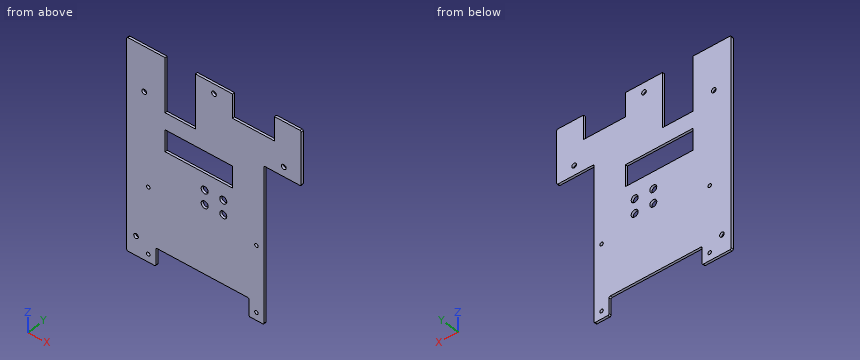
from build123d import *

# Parameters (mm, degrees)
CROQUIS1_W         = 150
CROQUIS1_H         = 175.2
CROQUIS1_R         = 1.5
EXTRUIR1_DEPTH     = 2
CROQUIS2_W         = 80
CROQUIS2_H         = 15
EXTRUIR2_DEPTH     = 10
CROQUIS3_W         = 32
CROQUIS3_H         = 130
EXTRUIR3_DEPTH     = 10
CROQUIS4_R         = 2
EXTRUIR4_DEPTH     = 10
CROQUIS5_R         = 3
EXTRUIR5_DEPTH     = 10
MATRIZL1_COUNT     = 2
MATRIZL1_PITCH     = 8
MATRIZL1_COL_COUNT = 2
MATRIZL1_COL_PITCH = 8
CROQUIS6_R         = 3
EXTRUIR6_DEPTH     = 2
CROQUIS7_W         = 26
CROQUIS7_H         = 45.2
CROQUIS7_W_2       = 36
CROQUIS7_H_2       = 20
CROQUIS7_W_3       = 58
CROQUIS7_H_3       = 18
EXTRUIR7_DEPTH     = 10
REDONDEO1_R        = 1


with BuildPart() as part:
    # Croquis1 → Extruir1 (new body)
    with BuildSketch(Plane(origin=(0, 0, 0), x_dir=(1, 0, 0), z_dir=(0, 1, 0))):
        Rectangle(CROQUIS1_W, CROQUIS1_H)
        with Locations(Location((-56.5, 81.1, 0), (0, 0, 270))):
            Circle(CROQUIS1_R, mode=Mode.SUBTRACT)
        with Locations(Location((36.5, 81.1, 0), (0, 0, 270))):
            Circle(CROQUIS1_R, mode=Mode.SUBTRACT)
        with Locations(Location((-56.5, 26.1, 0), (0, 0, 270))):
            Circle(CROQUIS1_R, mode=Mode.SUBTRACT)
        with Locations(Location((36.5, 26.1, 0), (0, 0, 270))):
            Circle(CROQUIS1_R, mode=Mode.SUBTRACT)
    extrude(amount=EXTRUIR1_DEPTH)

    # Croquis2 → Extruir2 (cut)
    with BuildSketch(Plane(origin=(0, 2, 0), x_dir=(1, 0, 0), z_dir=(0, 1, 0))):
        with Locations((-10, 80.1)):
            Rectangle(CROQUIS2_W, CROQUIS2_H)
    extrude(amount=-EXTRUIR2_DEPTH, mode=Mode.SUBTRACT)

    # Croquis3 → Extruir3 (cut)
    with BuildSketch(Plane(origin=(0, 2, 0), x_dir=(1, 0, 0), z_dir=(0, 1, 0))):
        with Locations((59, 22.6)):
            Rectangle(CROQUIS3_W, CROQUIS3_H)
    extrude(amount=-EXTRUIR3_DEPTH, mode=Mode.SUBTRACT)

    # Croquis4 → Extruir4 (cut)
    with BuildSketch(Plane(origin=(0, 2, 0), x_dir=(1, 0, 0), z_dir=(0, 1, 0))):
        with Locations(Location((-60, -50.4, 0), (0, 0, 270))):
            Circle(CROQUIS4_R)
        with Locations(Location((60, -50.4, 0), (0, 0, 270))):
            Circle(CROQUIS4_R)
        with Locations(Location((-67, 71.6, 0), (0, 0, 270))):
            Circle(CROQUIS4_R)
        with Locations(Location((0, -79.6, 0), (0, 0, 270))):
            Circle(CROQUIS4_R)
    extrude(amount=-EXTRUIR4_DEPTH, mode=Mode.SUBTRACT)

    # Croquis5 → Extruir5 (cut)
    with BuildSketch(Plane(origin=(0, 2, 0), x_dir=(1, 0, 0), z_dir=(0, 1, 0))):
        with Locations(Location((0, 15.6, 0), (0, 0, 270))):
            Circle(CROQUIS5_R)
        with Locations(Location((0, 3.6, 0), (0, 0, 270))):
            Circle(CROQUIS5_R)
    extruir5 = extrude(amount=-EXTRUIR5_DEPTH, mode=Mode.SUBTRACT)

    # MatrizL1: Extruir5 ×2
    with Locations(*[(-i * MATRIZL1_PITCH, 0, 0) for i in range(1, MATRIZL1_COUNT)]):
        add(extruir5, mode=Mode.SUBTRACT)

    # MatrizL1 col: Extruir5 ×2
    with Locations(*[(i * MATRIZL1_COL_PITCH, 0, 0) for i in range(1, MATRIZL1_COL_COUNT)]):
        add(extruir5, mode=Mode.SUBTRACT)

    # Croquis6 → Extruir6 (add)
    with BuildSketch(Plane(origin=(0, 2, 0), x_dir=(1, 0, 0), z_dir=(0, 1, 0))):
        with Locations((0, 15.6)):
            Circle(CROQUIS6_R)
        with Locations((0, 3.6)):
            Circle(CROQUIS6_R)
    extrude(amount=-EXTRUIR6_DEPTH)

    # Croquis7 → Extruir7 (cut)
    with BuildSketch(Plane(origin=(0, 2, 0), x_dir=(1, 0, 0), z_dir=(0, 1, 0))):
        with Locations((-29, -65)):
            Rectangle(CROQUIS7_W, CROQUIS7_H)
        with Locations((34, -77.6)):
            Rectangle(CROQUIS7_W_2, CROQUIS7_H_2)
        with Locations((-13, -19.4)):
            Rectangle(CROQUIS7_W_3, CROQUIS7_H_3)
    extrude(amount=-EXTRUIR7_DEPTH, mode=Mode.SUBTRACT)

    # Redondeo1
    redondeo1_edges = [part.edges().sort_by_distance(p)[0] for p in [
        (30, 1, -87.6),
        (-50, 1, -87.6),
        (30, 1, -72.6),
        (-50, 1, -72.6),
        (43, 1, -87.6),
        (75, 1, 42.4),
        (43, 1, 42.4),
        (-75, 1, -87.6),
        (75, 1, 87.6),
        (-75, 1, 87.6),
    ]]
    fillet(redondeo1_edges, radius=REDONDEO1_R)


solid = part.part
Source: CAD feature listing. Evaluate the final solid. Frame: model axes, mm. Round coordinates to 2 decimals unless told otherwise and drop trailing zeros. Loops run counter-clockwise (first coordinate to the right, second up) from the corner with the lowest first, then second, coordinate; pieces in that order, holes last.
Q1. Section A-A, the plane x = 0. Return loops of the section in (y, z), plus the area to 3 significant figures.
Q2. Section C-C, the plane x = -60. Return loops of the section in (y, z).
Q3. First-contact query: P1, Ø5, axis at x = 36.5, z = -81.1, coming from the +Y side; P2, Ø1, axis at x = 62, y = 1, coming from the -Z side. Flat tips, straight axial feed; report the tip coordinate or a pass-through.
Q4. Ray query, line 1 (X direction, y = 1.25, z = -81.1); line 2 (X direction, y = 0.9, z = -3.6); line 3 (Z direction, x = 7.5, y = 1.9). Return the intervals inside material, ascending.
Q5. Section B-B, the plane z = -15.6. Return loops of the section in (x, y).
Q6. Section D-D, the plane z = 65.5. Return loops of the section in (x, y), plus the area to 3 significant figures.
Solutions:
1. outline: (0, -72.6) - (2, -72.6) - (2, 10.4) - (0, 10.4) - close; (0, 28.4) - (2, 28.4) - (2, 77.6) - (0, 77.6) - close; (0, 81.6) - (2, 81.6) - (2, 87.6) - (0, 87.6) - close
1. area: 276 mm2
2. outline: (0, -87.6) - (2, -87.6) - (2, 48.4) - (0, 48.4) - close; (0, 52.4) - (2, 52.4) - (2, 87.6) - (0, 87.6) - close
3. P1: stops at y = 2
3. P2: stops at z = 42.4
4. line 1: x = -75 to -58, -55 to -50, 30 to 35, 38 to 43
4. line 2: x = -75 to -11, -5 to 5, 11 to 43
4. line 3: z = -72.6 to -18.56, -12.64 to -6.56, -0.64 to 10.4, 28.4 to 87.6
5. outline: (-75, 0) - (-11, 0) - (-11, 2) - (-75, 2) - close; (-5, 0) - (5, 0) - (5, 2) - (-5, 2) - close; (11, 0) - (43, 0) - (43, 2) - (11, 2) - close
6. outline: (-75, 0) - (-42, 0) - (-42, 2) - (-75, 2) - close; (-16, 0) - (75, 0) - (75, 2) - (-16, 2) - close
6. area: 248 mm2
